Answer from the drawing. Dimensions are ordinates in mm from the lowest x, y and z of the part. Round coordinates to 2 decimals unless told otherwise and drop trailing zeros. Write each loop counter-clockwise with the first axis right and the second up, starting at its lowest first coordinate (ties: lowest second). Pieces come first, ordered by that corner, then holes.
1. Straight lines are drawn through the part: probe 1 along Z at (x, y) = (183, 0.25); probe 2 along X at (y, z) = (0.75, 66). For each, find the intervals that lie inside material, in ascending order.
2. Find section C-C (y = 1.45). Write down the section's boundary in (x, z), and give its area (3 significant figures).
3. Find section A-A (z = 62.5). Write down the section's boundary in (x, y).
4. Find section B-B (x = 182.5). Write down the section's boundary in (y, z), and give its area (3 significant figures).
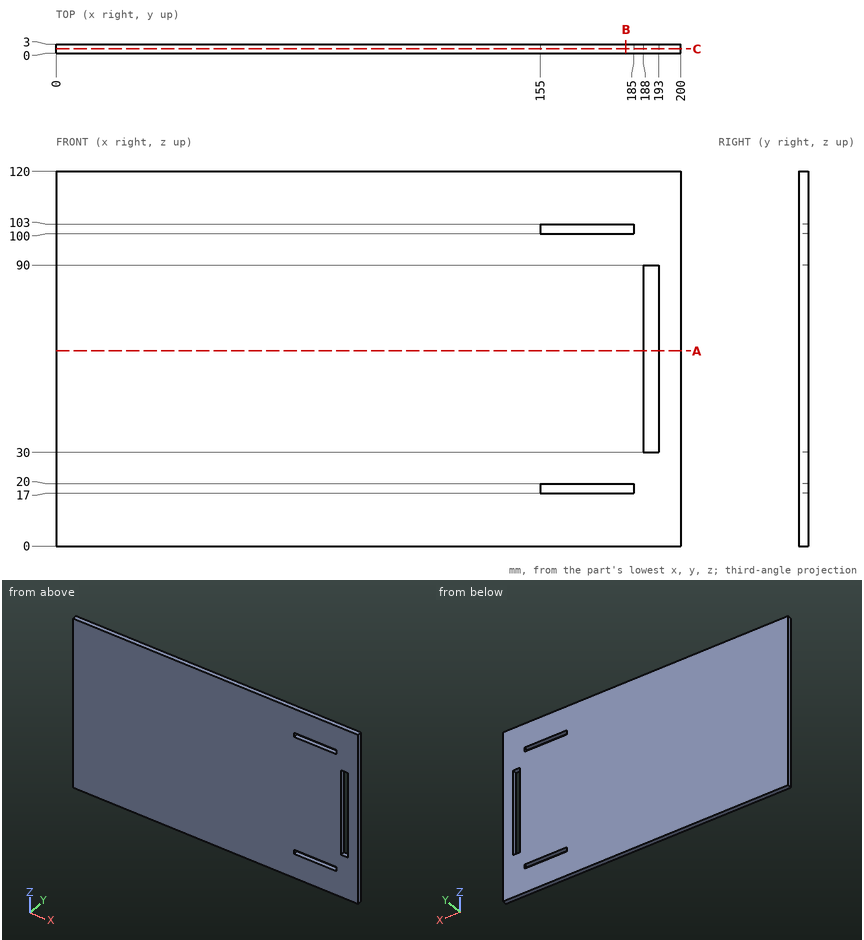
Worked answers:
1. probe 1: z = 0 to 17, 20 to 100, 103 to 120
1. probe 2: x = 0 to 188, 193 to 200
2. outline: (0, 0) - (200, 0) - (200, 120) - (0, 120) - close; hole (155, 17) - (185, 17) - (185, 20) - (155, 20) - close; hole (155, 100) - (185, 100) - (185, 103) - (155, 103) - close; hole (188, 30) - (193, 30) - (193, 90) - (188, 90) - close
2. area: 23,500 mm2
3. outline: (0, 0) - (188, 0) - (188, 3) - (0, 3) - close; (193, 0) - (200, 0) - (200, 3) - (193, 3) - close
4. outline: (0, 0) - (3, 0) - (3, 17) - (0, 17) - close; (0, 20) - (3, 20) - (3, 100) - (0, 100) - close; (0, 103) - (3, 103) - (3, 120) - (0, 120) - close
4. area: 342 mm2
